Source: three-view drawing plus pictorial views. Frame: mm from the lowest corner of the part. A direction names the side the tool comes from. Give positions to 0.01 mm unless a question says otherwise; leave off trailing zeros. Loops run counter-clockwise (first coordinate to the right, second up) from the corner with the lowest first, then second, coordinate; pieces in that order, holes last. Notation, with made-up numbers: (71.5, 65.5) - (118.5, 65.5) arc R18 cw to (118.5, 76.5) - close; hole circle Ø3 at (87, 28). An arc over 180 degrees is marked (long way). Put each result on its own line as item: value.
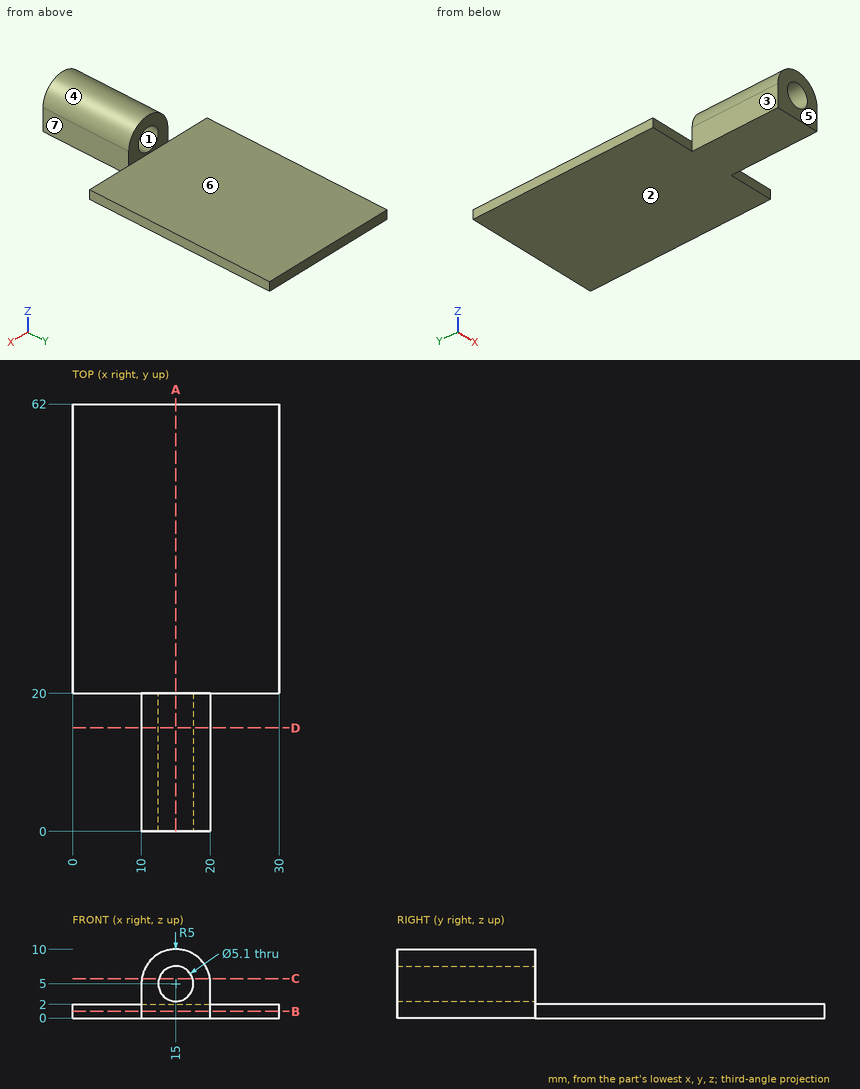
1) Section query D-D, the plane y = 15. Output: boundary loops of the cut face in (x, z).
Check result:
outline: (10, 0) - (20, 0) - (20, 5) arc R5 ccw to (10, 5) - close; hole circle Ø5.1 at (15, 5)
2) Section query B-B, the plane z = 1. Output: boundary loops of the cut face in (x, y), plus the area to 3 significant figures.
Check result:
outline: (0, 20) - (10, 20) - (10, 0) - (20, 0) - (20, 20) - (30, 20) - (30, 62) - (0, 62) - close
area: 1,460 mm²
3) Access query for the marked faces 5, 6 and 7. Directions: +Z, -Z, +X, -X, +Y, -Y. A direction counts if a zero-diameter tool reaches every point of the face in a straight line with its end or side. Return the directions, or none.
Check result:
face 5: +Z, -Z, +X, -X, -Y
face 6: +Z, +X, -X, +Y
face 7: +Z, -Z, +X, -Y
4) Pin query (flat end, axial travel): P1, Ø0.6, axis at x = 26, z = 1, coming from the -Y side; P2, Ø1.5, axis at y = 7.5, z = 8, coming from the +X side; P3, Ø5, axis at x = 15, z = 7.5, coming from the +Y side. Return the tip coordinate at first contact, or that it passes through.
Check result:
P1: y = 20
P2: x = 19.47
P3: y = 20
5) Mould query, pull axis Z, two halves, no side actions, for the marked faces 1, 2, 3 and 4. Classes: pulls with the +Z half, pulls with the -Z half, needs draft (parallel to the pull), parting line crosses it, or undercut.
Check result:
face 1: undercut
face 2: pulls with the -Z half
face 3: needs draft
face 4: pulls with the +Z half
6) Section query A-A, the plane x = 15. Output: boundary loops of the cut face in (y, z), plus the area to 3 significant figures.
Check result:
outline: (0, 0) - (62, 0) - (62, 2) - (20, 2) - (20, 2.45) - (0, 2.45) - close; (0, 7.55) - (20, 7.55) - (20, 10) - (0, 10) - close
area: 182 mm²
7) Section query C-C, the plane z = 5.75. Output: boundary loops of the cut face in (x, y).
Check result:
outline: (10.06, 0) - (12.56, 0) - (12.56, 20) - (10.06, 20) - close; (17.44, 0) - (19.94, 0) - (19.94, 20) - (17.44, 20) - close
8) Material intervals for line 1 along Z through (x, y) = (15, 10); line 2 along Z through (x, y) = (19, 22); line 3 along Z through (x, y) = (14.25, 3.5), sorted ascending. Write a range as [from, to].
Check result:
line 1: [0, 2.45], [7.55, 10]
line 2: [0, 2]
line 3: [0, 2.56], [7.44, 9.94]
